Geometry: final body of the model. Coordinates: model frame, mm. Face numbers are marked on the shaded views. A direction names the side the tool comes from. Give positions to 0.01 mm unless a question says otherwise; leave off trailing zeros. Write each loop counter-clockwise with the first axis right and the second up, starting at its lowest first coordinate (ties: lowest second). Pieces come first, ordered by that corner, then holes. Notation, with made-up numbers: M 87.5,68 L 97.5,68 A17 ccw 97.5,79 Z; hole C -40,49 d4. An arc over 180 degrees is marked long. Use a Markdown table: item, result. Add a question column.
(1) Draft query along Z for the marked faces 3, 4 and 5. Return one class per face: released by +Z, released by -Z, zero draft, split by the parting line, or undercut.
(2) Reachability of the marked faces 1 and 2 from +Z, -Z, +X, -X, +Y, -Y: full face, straight path, thin tool, end or side. Return the list, or none.
(3) Material intervals for L1, parallel to Z at x = -15.5, y = 15; L2, parallel to X at y = 10.25, z = 19; L3, parallel to Z at x = 28.5, y = 6.75, sorted ascending.
(4) Cut plane C-C (z = 6.5). Output: boundary loops of the cut face in (x, y), plus the area to 3 significant figures.
(5) Cut plane D-D (y = 5.5). Output: boundary loops of the cut face in (x, z), plus the area to 3 significant figures.
(6) Cut plane B-B (y = 14.25). Output: boundary loops of the cut face in (x, z).
(7) Pin query (flat end, axial travel): pin 1 Ø4 at (x, z) = (2.5, -6.5) entering from +Y (3 decimals); pin 2 Ø3 at (x, z) = (16.5, -5.5) entering from +Y. Return the tip coordinate at first contact, or that it passes through.
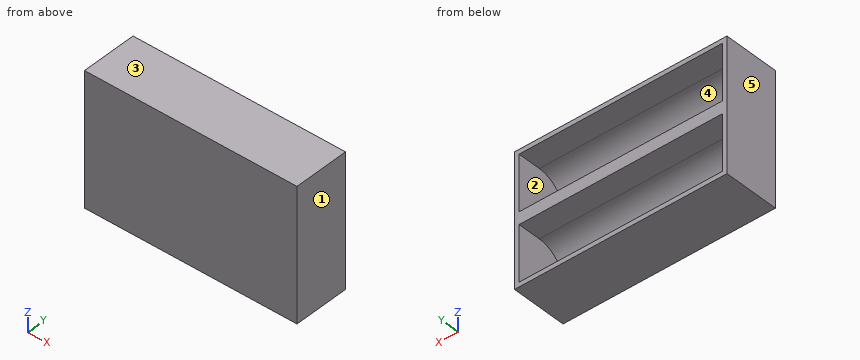
Autodesk Inventor part; units mm, degrees
ref_plane "YZ Plane" through (0, 0, 0) normal (1, 0, 0) x (0, 1, 0)
ref_plane "XZ Plane" through (0, 0, 0) normal (0, 1, 0) x (-1, 0, 0)
ref_plane "XY Plane" through (0, 0, 0) normal (0, 0, 1) x (1, 0, 0)
sketch "Sketch1" plane through (0, 0, 0) normal (0, 1, 0) x (-1, 0, 0)
  line L0 (33, 20) -> (-33, 20)
  line L1 (-33, 20) -> (-33, -20)
  line L2 (-33, -20) -> (33, -20)
  line L3 (33, -20) -> (33, 20)
  line L4 (33, 2) -> (-33, 2)
  line L5 (33, -2) -> (-33, -2)
  line L6 (-34.5, 21.5) -> (34.5, 21.5)
  line L7 (34.5, 21.5) -> (34.5, -21.5)
  line L8 (34.5, -21.5) -> (-34.5, -21.5)
  line L9 (-34.5, -21.5) -> (-34.5, 21.5)
  point P0 (0, 0)
  dimension "d0" = 66
  dimension "d1" = 33
  dimension "d2" = 40
  dimension "d3" = 20
  dimension "d4" = 18
  dimension "d5" = 18
  dimension "d6" = 1.5
extrude "Extrusion1" add sketch "Sketch1" along normal blind 1.5 contours L3 L4 L1 L0 | L3 L5 L1 L4 | L3 L2 L1 L5 | L6 L7 L8 L9
sketch "Sketch2" plane through (0, 1.5, 0) normal (0, 1, 0) x (1, 0, 0)
  point P0 (0, 0)
extrude "Extrusion2" add sketch "Sketch1" along normal blind 18 contours L3 L5 L1 L4 | L6 L7 L8 L9
fillet "Fillet1" radius 9 4 edges at (0, 1.5, 2) (0, 1.5, 20) (0, 1.5, -2) (0, 1.5, -20)
properties part number "battery rack"
Answer list:
| question | item | result |
|---|---|---|
| 1 | face 3 | released by +Z |
| 1 | face 4 | undercut |
| 1 | face 5 | zero draft |
| 2 | face 1 | +Z, -Z, +X, +Y, -Y |
| 2 | face 2 | +Y |
| 3 | L1 | -21.5 to -20, -2 to 2, 20 to 21.5 |
| 3 | L2 | -34.5 to -33, 33 to 34.5 |
| 3 | L3 | -21.5 to -19.18, -2.82 to 2.82, 19.18 to 21.5 |
| 4 | outline | M -34.5,0 L 34.5,0 L 34.5,18 L 33,18 L 33,2.71 L -33,2.71 L -33,18 L -34.5,18 Z |
| 4 | area | 233 mm² |
| 5 | outline | M -34.5,-21.5 L 34.5,-21.5 L 34.5,21.5 L -34.5,21.5 Z; hole M -33,-18.48 L 33,-18.48 L 33,-3.52 L -33,-3.52 Z; hole M -33,3.52 L 33,3.52 L 33,18.48 L -33,18.48 Z |
| 5 | area | 991 mm² |
| 6 | outline | M -34.5,-21.5 L 34.5,-21.5 L 34.5,21.5 L -34.5,21.5 Z; hole M -33,-20 L 33,-20 L 33,-2 L -33,-2 Z; hole M -33,2 L 33,2 L 33,20 L -33,20 Z |
| 7 | pin 1 | y = 4.275 |
| 7 | pin 2 | y = 4.84 |
